Answer from the drawing. Dimensions are ordinates in mm from the lowest x, y and z of the part. A direction names the side the tool comes from. Coordinates: 2 decimals unless noted, no trailing zeros. Write each loop counter-clockwise with the first axis right and the second up, starting at its lowest first coordinate (ties: lowest second). Pieces come first, ordered by that corner, then holes.
1) Find the intervals of material crossed by line 1 (Z direction, x = 2.5, y = 1.45); line 2 (X direction, y = 1.2, z = 25); line 3 (X direction, y = 1.65, z = 21.5), in increasing order.
2) Each of these flat-tipped pins is pushed along its axis until it touches: pin 1 Ø0.9 at (y, z) = (1, 7.5) entering from -X; pin 2 Ø1.5 at (y, z) = (1, 15) entering from +X; pin 3 Ø0.9 at (x, y) = (1.5, 1.5) entering from -Z. Where does it stop, or does it pass through?
3) The part is cut by section A-A (x = 12). Determine the outline of the cut face in (y, z), then the cut area to 3 significant figures.
4) The part is cut by section D-D (x = 1). Determine the outline of the cut face in (y, z), then the cut area to 3 significant figures.
5) The part is cut by section C-C (z = 26). Determine the outline of the cut face in (x, y), then the cut area to 3 significant figures.
6) Which of the six approach directions +Z, -Z, +X, -X, +Y, -Y give full straight-line access (tool end or side, diameter ignored) to the marked faces 1, 2 and 3?
7) The part is cut by section B-B (y = 1.15). Determine the outline of the cut face in (x, z), then the cut area to 3 significant figures.
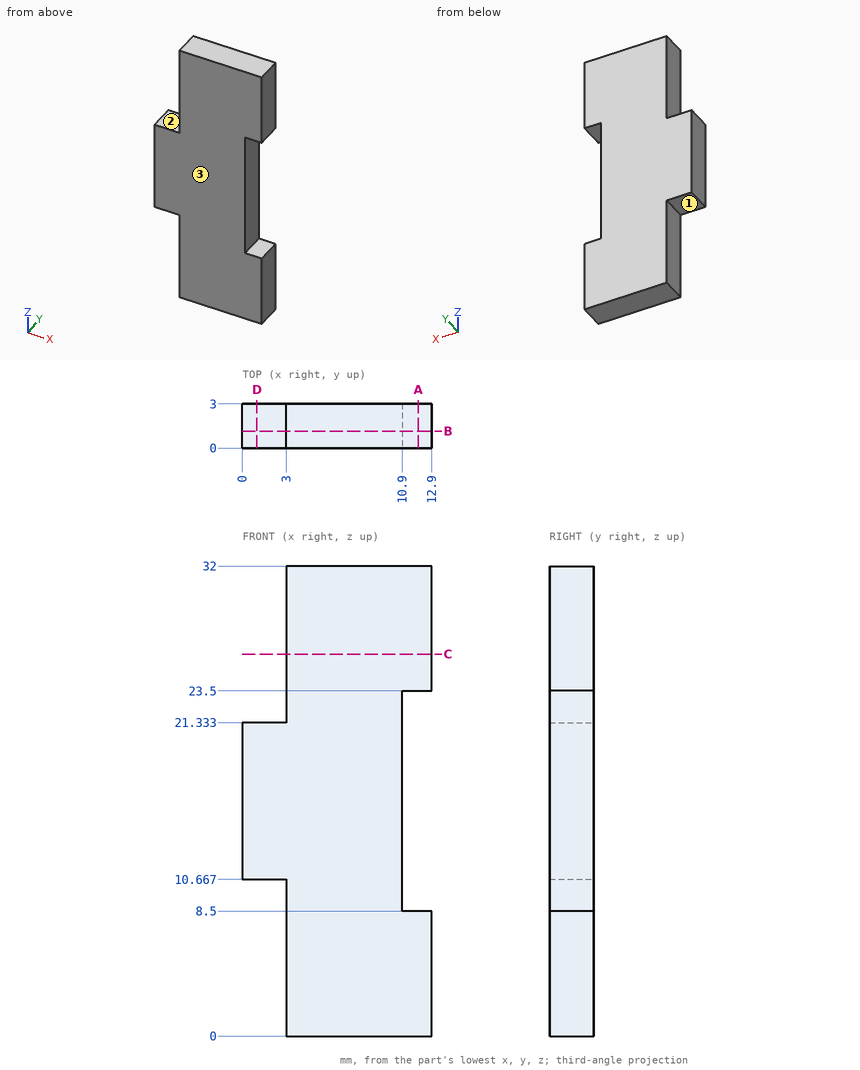
Reported:
1. line 1: z = 10.67 to 21.33
1. line 2: x = 3 to 12.9
1. line 3: x = 3 to 10.9
2. pin 1: stops at x = 3
2. pin 2: stops at x = 10.9
2. pin 3: stops at z = 10.67
3. outline: (0, 0) - (3, 0) - (3, 8.5) - (0, 8.5) - close; (0, 23.5) - (3, 23.5) - (3, 32) - (0, 32) - close
3. area: 51.0 mm2
4. outline: (0, 10.67) - (3, 10.67) - (3, 21.33) - (0, 21.33) - close
4. area: 32.0 mm2
5. outline: (3, 0) - (12.9, 0) - (12.9, 3) - (3, 3) - close
5. area: 29.7 mm2
6. face 1: -Z, -X, +Y, -Y
6. face 2: +Z, -X, +Y, -Y
6. face 3: +Z, -Z, +X, -X, -Y
7. outline: (0, 10.67) - (3, 10.67) - (3, 0) - (12.9, 0) - (12.9, 8.5) - (10.9, 8.5) - (10.9, 23.5) - (12.9, 23.5) - (12.9, 32) - (3, 32) - (3, 21.33) - (0, 21.33) - close
7. area: 319 mm2
